Geometry: final body of the model. Coordinates: model frame, mm. A direction names the side the tool comes from. Round coordinates to 2 decimals unless told otherwise and drop trailing zeros. Loops run counter-clockwise (first coordinate to the right, second up) from the corner with the lowest first, then second, coordinate; pieces in that order, holes last. Notation, with made-up numbers: M 64,-26 L 72,-26 A18 cw 72,-18 Z; hole C 18.5,-7 d3. An arc over 180 degrees is marked long. Answer as a JSON object with one key per item and string values.
from build123d import *

# Parameters (mm, degrees)
SKETCH1_R           = 101.6
BOSS_EXTRUDE1_DEPTH = 6.35


with BuildPart() as part:
    # Sketch1 → Boss-Extrude1 (new body)
    with BuildSketch(Plane.XY):
        Circle(SKETCH1_R)
        with BuildLine():
            Line((-12.7, 14.199031657), (-12.7, 75.134213245))
            ThreePointArc((-12.7, 75.134213245), (-65.991135768, 38.1), (-71.418137364, -26.568583995))
            Line((-71.418137364, -26.568583995), (-18.646722124, 3.8990068))
            ThreePointArc((-18.646722124, 3.8990068), (-16.497783942, 9.525), (-12.7, 14.199031657))
        make_face(mode=Mode.SUBTRACT)
        with BuildLine():
            Line((12.7, 14.199031657), (12.7, 75.134213245))
            ThreePointArc((12.7, 75.134213245), (65.991135768, 38.1), (71.418137364, -26.568583995))
            Line((71.418137364, -26.568583995), (18.646722124, 3.8990068))
            ThreePointArc((18.646722124, 3.8990068), (16.497783942, 9.525), (12.7, 14.199031657))
        make_face(mode=Mode.SUBTRACT)
        with BuildLine():
            Line((5.946722124, -18.098038457), (58.718137364, -48.565629251))
            ThreePointArc((58.718137364, -48.565629251), (0, -76.2), (-58.718137364, -48.565629251))
            Line((-58.718137364, -48.565629251), (-5.946722124, -18.098038457))
            ThreePointArc((-5.946722124, -18.098038457), (0, -19.05), (5.946722124, -18.098038457))
        make_face(mode=Mode.SUBTRACT)
    extrude(amount=BOSS_EXTRUDE1_DEPTH)


solid = part.part
1) Pull-direction query (X, two-part tool) for faces 1 (the flat face through (-1, 1, 0)), 2 (the cylindrical face through (65.517, 38.91, 3.131)), 3 (the cylindrical face through (-22.025, -99.184, 3.131)); classes: +X half, -X half, draft (parallel to the pull), parting line (faces both ways), or undercut.
Results:
{"face 1": "draft", "face 2": "undercut", "face 3": "parting line"}
2) Pin query (flat end, axial travel): P1, Ø3, axis at y = 61, z = 2, coming from the -X side; P2, Ø4, axis at x = -15.5, y = 37, coming from the -Z side; P3, Ø2, axis at x = -7, z = 4.5, coming from the +Y side; P4, Ø3, axis at y = 40, z = 4.5, coming from the -X side. Return the tip coordinate at first contact, or that it passes through.
Results:
{"P1": "x = -82.35", "P2": "through", "P3": "y = 101.42", "P4": "x = -94.02"}
3) Section query A-A (x = 0). Return the cut outline in (y, z), and give its area (3 significant figures).
Results:
{"outline": "M -101.6,0 L -76.2,0 L -76.2,6.35 L -101.6,6.35 Z; M -19.05,0 L 101.6,0 L 101.6,6.35 L -19.05,6.35 Z", "area": "927 mm2"}
4) Section query C-C (z = 1). Return the cut outline in (x, y).
Results:
{"outline": "C 0,0 d203.2; hole M -71.42,-26.57 L -18.65,3.9 A19.05 cw -12.7,14.2 L -12.7,75.13 A76.2 ccw Z; hole M -58.72,-48.57 A76.2 ccw 58.72,-48.57 L 5.95,-18.1 A19.05 cw -5.95,-18.1 Z; hole M 12.7,14.2 A19.05 cw 18.65,3.9 L 71.42,-26.57 A76.2 ccw 12.7,75.13 Z"}
5) Section query B-B (y = 20). Return the cut outline in (x, z), and give its area (3 significant figures).
Results:
{"outline": "M -99.61,0 L -73.53,0 L -73.53,6.35 L -99.61,6.35 Z; M -12.7,0 L 12.7,0 L 12.7,6.35 L -12.7,6.35 Z; M 73.53,0 L 99.61,0 L 99.61,6.35 L 73.53,6.35 Z", "area": "493 mm2"}
6) Section query D-D (y = -30). Return the cut outline in (x, z), and give its area (3 significant figures).
Results:
{"outline": "M -97.07,0 L -26.56,0 L -26.56,6.35 L -97.07,6.35 Z; M 26.56,0 L 97.07,0 L 97.07,6.35 L 26.56,6.35 Z", "area": "895 mm2"}
7) Reachability of faces 4 (the flat face through (12.7, 44, 3)), 5 (the flat face through (-1, 1, 6.35)) from +Z, -Z, +X, -X, +Y, -Y: full face, straight path, thin tool, end or side. Return the list, or none.
Results:
{"face 4": "+Z, -Z", "face 5": "+Z, +X, -X, +Y, -Y"}
8) Ray query, line 1 (Y direction, x = -41, z = 2.5); line 2 (X direction, y = 23, z = 4); line 3 (X direction, y = 10.5, z = 1.5). Return the intervals inside material, ascending.
Results:
{"line 1": "-92.96 to -64.23, -38.34 to -9.01, 64.23 to 92.96", "line 2": "-98.96 to -72.65, -12.7 to 12.7, 72.65 to 98.96", "line 3": "-101.06 to -75.47, -15.9 to 15.9, 75.47 to 101.06"}
